Verification items for the finished model (mm, model axes). Give positions to 0.01 mm unless a question says otherwise; leave off trailing zeros. Order: outer loops, then holes, each group sorted by start corner. A loop starts at its lowest first (then second) coordinate and runs counter-clockwise, first axis right, second up. Notation, with made-up numbers: (58, 55) - (89, 55) arc R29 cw to (89, 76) - close; hole circle Ø1 at (72, 14). An arc over 180 degrees is marked (long way). Answer as a JSON object with one key per item and string values.
Solid Edge part; units mm, degrees
sketch "Sketch1" plane through (0, 0, 0) normal (1, 0, 0) x (0, 1, 0)
  line L0 (27.5, -27) -> (27.5, 15.5)
  line L1 (27.5, 15.5) -> (-27.5, 15.5)
  line L2 (-27.5, 15.5) -> (-27.5, -27)
  line L3 (-27.5, -27) -> (27.5, -27)
extrude "Protrusion1" add sketch "Sketch1" along normal blind 2
sketch "Sketch2" plane through (0, 0, 0) normal (1, 0, 0) x (0, 1, 0)
  circle A0 centre (0, 10) radius 1.6
  circle A1 centre (19, -14) radius 1.6
extrude "ExtrudedCutout_7" cut sketch "Sketch2" along normal blind 2
properties material "ABS Plastic, high impact"
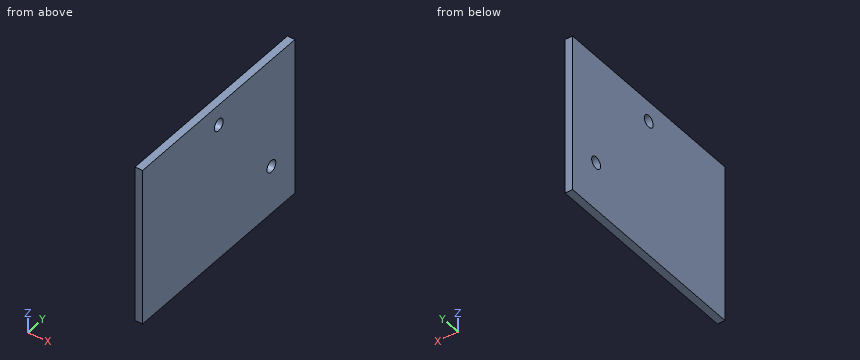
(1) Section check A-A (z = -14). Record the cut outline in (x, y).
Computed values:
{"outline": "(0, -27.5) - (2, -27.5) - (2, 17.4) - (0, 17.4) - close; (0, 20.6) - (2, 20.6) - (2, 27.5) - (0, 27.5) - close"}
(2) Material ranges on line 1 along Z through (x, y) = (1.2, 0); line 2 along Z through (x, y) = (0.7, 19); line 3 along Y through (x, z) = (1.6, 10.5), recorded low to high. Write a range as [from, to].
Computed values:
{"line 1": "z = [-27, 8.4], [11.6, 15.5]", "line 2": "z = [-27, -15.6], [-12.4, 15.5]", "line 3": "y = [-27.5, -1.52], [1.52, 27.5]"}
(3) Section check B-B (y = 19). Record the cut outline in (x, z), then the cut area to 3 significant figures.
Computed values:
{"outline": "(0, -27) - (2, -27) - (2, -15.6) - (0, -15.6) - close; (0, -12.4) - (2, -12.4) - (2, 15.5) - (0, 15.5) - close", "area": "78.6 mm²"}
